Design review of the part built by this model. Coordinates are the model's own, in mm. Face numbers are marked on the shaded views. A direction names the side the tool comes from. Give positions to 0.01 mm unless a question says otherwise; leave off trailing zeros. Order: outer loops, then holes, each group sorted by start corner. A loop starts at its lowest first (then second) coordinate and runs counter-clockwise, first axis right, second up. Notation, with made-up numbers: (53.25, 41.5) -> (112.25, 41.5) arc R22 cw to (112.25, 64.5) -> close; hole circle Ø11 at (48, 13.25). An arc over 180 degrees is marked (long way). One line per item, written item: value. Start each with the question number.
1) Consider section A-A (x = 31.5). State the section outline as (y, z) points, plus the area to 3 significant figures.
2) Tool access review of the marked faces 4 and 5: name each direction out of +Z, -Z, +X, -X, +Y, -Y from which nothing blocks a thin tool from reaching the whole face with its end or side.
3) Consider section B-B (y = 4.25). State the section outline as (x, z) points, plus the area to 3 significant figures.
4) The part is to be moulded in two halves that separate along X. For the marked faces 1, 2 and 3, say which applies: released by +X, released by -X, zero draft, split by the parting line, or undercut.
5) Wall thickness on line 1 along Y through (x, z) = (31.5, 2.3); line 2 along Y through (x, z) = (-18, 1); line 3 along X through (y, z) = (1, 3.25): over which ranges is each line inside the solid? List them lowest first. Write a range as from..to.
6) For pin 1 (1 mm diameter, centred on y = 1, z = 2.5, fed in from +X); pin 2 (1 mm diameter, centred on x = -3.5, z = 2, fed in from +Y), all flat-tipped, find the tip position at first contact; note any pin that passes through.
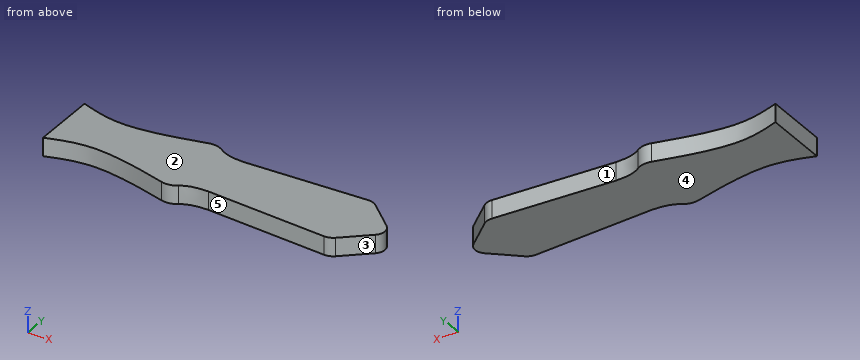
from build123d import *

# Parameters (mm, degrees)
F1_DEPTH = 4


with BuildPart() as f1:
    # F0 (on Top) → F1 (new body)
    with BuildSketch(Plane.XY):
        with BuildLine():
            Line((33.1839122816, 7.4341704185), (7, 6.0167759657))
            add(Edge.make_bspline(
                [(7, 6.0167759657), (4.0042999393, 6.0167759657), (2.4851097846, 6.5339730516), (1.3114110288, 7.3480597034)],
                knots=[0, 0, 0, 0, 5.2976431113, 5.2976431113, 5.2976431113, 5.2976431113], degree=3))
            ThreePointArc((1.3114110288, 7.3480597034), (-0.2690563082, 7.9996972089), (-1.9772483015, 7.9319583269))
            add(Edge.make_bspline(
                [(-1.9772483015, 7.9319583269), (-8.0874424423, 6.3392692714), (-18.8504021756, 3.7391038399), (-25.5343435285, 5.9978133829), (-28.5, 7)],
                knots=[0.0565322181, 0.0565322181, 0.0565322181, 0.0565322181, 0.5813845177, 1, 1, 1, 1], degree=3))
            Line((-28.5, 7), (-28.5, 0))
            Line((-28.5, 0), (-28.5, -7))
            add(Edge.make_bspline(
                [(-1.9772483015, -7.9319583269), (-8.0874424423, -6.3392692714), (-18.8504021756, -3.7391038399), (-25.5343435285, -5.9978133829), (-28.5, -7)],
                knots=[0.0565322181, 0.0565322181, 0.0565322181, 0.0565322181, 0.5813845177, 1, 1, 1, 1], degree=3))
            ThreePointArc((-1.9772483015, -7.9319583269), (-0.2690563082, -7.9996972089), (1.3114110288, -7.3480597034))
            add(Edge.make_bspline(
                [(7, -6.0167759657), (4.0042999393, -6.0167759657), (2.4851097846, -6.5339730516), (1.3114110288, -7.3480597034)],
                knots=[0, 0, 0, 0, 5.2976431113, 5.2976431113, 5.2976431113, 5.2976431113], degree=3))
            Line((7, -6.0167759657), (33.1839122816, -7.4341704185))
            ThreePointArc((33.1839122816, -7.4341704185), (34.3226011035, -7.2751722198), (35.3178602471, -6.6995404822))
            Line((35.3178602471, -6.6995404822), (40.8395039416, -1.8841535393))
            ThreePointArc((40.8395039416, -1.8841535393), (41.6963467853, 0), (40.8395039416, 1.8841535393))
            Line((40.8395039416, 1.8841535393), (35.3178602471, 6.6995404822))
            ThreePointArc((35.3178602471, 6.6995404822), (34.3226011035, 7.2751722198), (33.1839122816, 7.4341704185))
        make_face()
    extrude(amount=F1_DEPTH)


solid = f1.part
Checked values:
1. outline: (-7.34, 0) -> (7.34, 0) -> (7.34, 4) -> (-7.34, 4) -> close
1. area: 58.7 mm^2
2. face 4: -Z, +X, -X, +Y, -Y
2. face 5: +Z, -Z, -Y
3. outline: (-28.5, 0) -> (38.13, 0) -> (38.13, 4) -> (-28.5, 4) -> close
3. area: 267 mm^2
4. face 1: undercut
4. face 2: zero draft
4. face 3: released by +X
5. line 1: y = -7.34..7.34
5. line 2: y = -4.95..4.95
5. line 3: x = -28.5..41.49
6. pin 1: stops at x = 41.65
6. pin 2: stops at y = 7.67
